from build123d import *

# Parameters (mm, degrees)
SKETCH1_W           = 68.58
SKETCH1_H           = 53.34
BOSS_EXTRUDE1_DEPTH = 2.54
SKETCH2_W           = 12.7
SKETCH2_H           = 15.24
SKETCH2_W_2         = 3.39503639
SKETCH2_H_2         = 11.2855496
BOSS_EXTRUDE2_DEPTH = 5.08
SKETCH3_R           = 1.5875
CUT_EXTRUDE1_DEPTH  = 10.16
CUT_EXTRUDE2_DEPTH  = 3.54


with BuildPart() as part:
    # Sketch1 → Boss-Extrude1 (new body)
    with BuildSketch(Plane.XY):
        Rectangle(SKETCH1_W, SKETCH1_H)
    extrude(amount=BOSS_EXTRUDE1_DEPTH)

    # Sketch2 → Boss-Extrude2 (add)
    with BuildSketch(Plane.XY.offset(2.54)):
        with Locations((-34.29, 12.7)):
            Rectangle(SKETCH2_W, SKETCH2_H)
        with Locations((-34.29, -18.328779787)):
            Rectangle(SKETCH2_W_2, SKETCH2_H_2)
    extrude(amount=BOSS_EXTRUDE2_DEPTH)

    # Sketch3 → Cut-Extrude1 (cut)
    with BuildSketch(Plane.XY.offset(2.54)):
        with Locations((-19.05, 24.13)):
            Circle(SKETCH3_R)
        with Locations((-20.32, -24.13)):
            Circle(SKETCH3_R)
        with Locations((31.75, 8.89)):
            Circle(SKETCH3_R)
        with Locations((31.75, -19.05)):
            Circle(SKETCH3_R)
    extrude(amount=-CUT_EXTRUDE1_DEPTH, mode=Mode.SUBTRACT)

    # Sketch4 → Cut-Extrude2 (cut, through all)
    with BuildSketch(Plane.XY.offset(2.54)):
        Polygon((30.313159021, 26.67), (31.75, 25.233159021), (31.75, 13.012702255), (34.29, 11.115796447), (34.29, 26.67), align=None)
        Polygon((34.29, -23.181547096), (31.75, -25.078452904), (31.75, -26.67), (34.29, -26.67), align=None)
    extrude(amount=-CUT_EXTRUDE2_DEPTH, mode=Mode.SUBTRACT)


solid = part.part
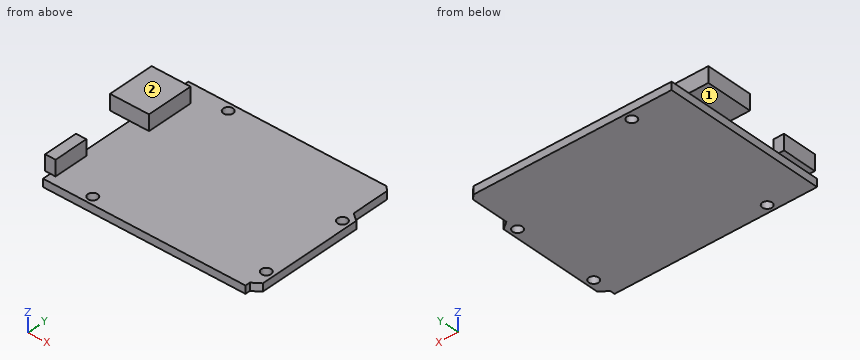
For this review, take the finished solid that the model builds, in its own axes (mm). Face numbers are marked on the shaded views. A direction names the side the tool comes from. Give positions to 0.01 mm unless a question says otherwise; leave off trailing zeros. Loops run counter-clockwise (first coordinate to the right, second up) from the corner with the lowest first, then second, coordinate; pieces in that order, holes last. Notation, with made-up numbers: (19.5, -6) - (30.5, -6) arc R19 ccw to (30.5, 12) - close; hole circle Ø5 at (-13, 71). An arc over 180 degrees is marked (long way). Write each question's results on one line, items separated by ' | '.
(1) For pin 1 Ø0.8 at (x, y) = (-35.5, -16) entering from -Z; pin 2 Ø2.5 at (y, z) = (-21, 4.5) entering from -X; pin 3 Ø2.5 at (y, z) = (12, 5) entering from +X, all flat-tipped, find the tip position at first contact; note any pin that passes through.
Conclusion:
pin 1: z = 2.54 | pin 2: x = -35.99 | pin 3: x = -27.94
(2) For the marked faces 1 and 2, list the 3-axis set-ups (+Z, -Z, +X, -X, +Y, -Y) from which the entire face can be reached by the end or side of a thin tool; tool diameter is ignored.
Conclusion:
face 1: -Z, -X, +Y, -Y | face 2: +Z, +X, -X, +Y, -Y
(3) Take a section at B-B (y = 8.89). Give the boundary of the cut face in (x, z).
Conclusion:
outline: (-40.64, 2.54) - (-34.29, 2.54) - (-34.29, 0) - (30.16, 0) - (30.16, 2.54) - (-27.94, 2.54) - (-27.94, 7.62) - (-40.64, 7.62) - close; (33.34, 0) - (34.29, 0) - (34.29, 2.54) - (33.34, 2.54) - close
(4) Take a section at C-C (x = -31). Give the boundary of the cut face in (y, z), then the cut area to 3 significant figures.
Conclusion:
outline: (-26.67, 0) - (26.67, 0) - (26.67, 2.54) - (20.32, 2.54) - (20.32, 7.62) - (5.08, 7.62) - (5.08, 2.54) - (-26.67, 2.54) - close | area: 213 mm^2
(5) Take a section at A-A (z = 5). Give the boundary of the cut face in (x, y).
Conclusion:
outline: (-40.64, 5.08) - (-27.94, 5.08) - (-27.94, 20.32) - (-40.64, 20.32) - close; (-35.99, -23.97) - (-32.59, -23.97) - (-32.59, -12.69) - (-35.99, -12.69) - close
(6) Take a section at D-D (y = -14). Give the boundary of the cut face in (x, z), then the cut area to 3 significant figures.
Conclusion:
outline: (-35.99, 2.54) - (-34.29, 2.54) - (-34.29, 0) - (34.29, 0) - (34.29, 2.54) - (-32.59, 2.54) - (-32.59, 7.62) - (-35.99, 7.62) - close | area: 191 mm^2
(7) For line 1 along Y through (x, z) = (-19.05, 1.2); line 2 along Y through (x, z) = (-20.32, 0.6); line 3 along X through (y, z) = (-19, 2), list the stretches that pass through material, from the lowest coordinate up.
Conclusion:
line 1: -26.67 to -25.08, -23.18 to 22.54, 25.72 to 26.67 | line 2: -26.67 to -25.72, -22.54 to 23.18, 25.08 to 26.67 | line 3: -34.29 to 30.16, 33.34 to 34.29
